The listing builds one solid part. Answer for the finished solid, in the listing's coordinates (mm). Coordinates: 2 decimals unless noted, no trailing zeros. Loops run counter-clockwise (first coordinate to the right, second up) from the corner with the lowest first, then second, coordinate; pieces in that order, holes last. Notation, with made-up numbers: M 25,-15 L 69,-15 A26 ccw 69,17 Z; hole C 14,-13 d5. An arc over 180 degrees is marked long. Return JSON: item names as keys, results as strings. Group by question number.
1. Given P1, Ø1, axis at x = 47.5, z = 345, coming from the -Y side; P2, Ø1, axis at x = 107, z = 347.5, coming from the -Y side, each flat-ended and moving along its own axis, determine where each tip first touches the part or whether it passes through.
2. Section A-A (x = 55) is taken. Write down the section's boundary in (y, z), then the cut area to 3 significant figures.
3. Straight lines are drawn through the part: L1, parallel to X at y = -337.5, z = 346; L2, parallel to X at y = -338.5, z = 343.75; L3, parallel to X at y = -341.5, z = 348.5. For each, find the intervals that lie inside material, in ascending order. Write a range as from..to.
Autodesk Inventor part; units mm, degrees
ref_plane "YZ Plane" through (0, 0, 0) normal (1, 0, 0) x (0, 1, 0)
ref_plane "XZ Plane" through (0, 0, 0) normal (0, 1, 0) x (-1, 0, 0)
ref_plane "XY Plane" through (0, 0, 0) normal (0, 0, 1) x (1, 0, 0)
sketch "Skizze2" plane through (0, 0, 0) normal (1, 0, 0) x (0, 1, 0)
  line L0 (-333.777, 348.0872) -> (-334.0423, 350.6737)
  line L1 (-333.777, 348.0872) -> (-333.134, 341.8201)
  line L2 (-333.134, 341.8201) -> (-342.5844, 340.8506)
  line L3 (-342.0005, 349.8573) -> (-334.0423, 350.6737)
  line L4 (-342.7069, 342.0444) -> (-341.2147, 342.1975)
  line L5 (-342.7069, 342.0444) -> (-342.5844, 340.8506)
  line L6 (-333.134, 341.8201) -> (-342.5844, 340.8506)
  line L7 (-333.777, 348.0872) -> (-333.134, 341.8201)
  line L8 (-333.777, 348.0872) -> (-341.7352, 347.2708)
  line L9 (-341.2147, 342.1975) -> (-341.7352, 347.2708)
  line L10 (-342.7069, 342.0444) -> (-342.5844, 340.8506)
  line L11 (-341.7352, 347.2708) -> (-342.0005, 349.8573)
  point P0 (0, 0)
extrude "Extrusion1" add sketch "Skizze2" along normal blind 69.4
sketch "Skizze3" plane through (0, 0, 0) normal (-1, 0, 0) x (0, 0, 1)
  line L0 (342.0444, -342.7069) -> (342.1975, -341.2147)
  line L1 (342.0444, -342.7069) -> (340.8506, -342.5844)
  line L2 (341.8201, -333.134) -> (340.8506, -342.5844)
  line L3 (348.0872, -333.777) -> (341.8201, -333.134)
  line L4 (348.0872, -333.777) -> (347.2708, -341.7352)
  line L5 (342.1975, -341.2147) -> (347.2708, -341.7352)
  line L6 (350.6737, -334.0423) -> (349.8573, -342.0005)
  line L7 (349.8573, -342.0005) -> (347.2708, -341.7352)
  line L8 (349.8573, -342.0005) -> (342.1975, -341.2147)
  line L9 (341.8201, -333.134) -> (350.6737, -334.0423)
  line L10 (350.6737, -334.0423) -> (348.0872, -333.777)
  point P0 (0, 0)
extrude "Extrusion2" cut sketch "Skizze3" against normal blind 10 contours L4 L9 L6 L7
sketch "Skizze4" plane through (0, -333.134, 341.8201) normal (0, 0.1020498, -0.9947793) x (1, 0, 0)
  line L0 (5, 0) -> (5, 9.5) construction
  line L1 (0, 9.5) -> (69.4, 9.5) construction
  circle A0 centre (5, 4) radius 2.85
  circle A1 centre (5, 4) radius 1.5 construction
  point P0 (0, -296.5122)
  dimension "d4" = 5.7
extrude "Extrusion3" cut sketch "Skizze4" against normal blind 3.1
sketch "Skizze5" plane through (5, -337.4295, 344.4957) normal (0, 0.1020498, -0.9947793) x (-1, 0, 0)
  circle A0 centre (0, 0) radius 2.85
  circle A1 centre (0, 0) radius 1.5
  point P0 (5, 300.5122)
  dimension "d9" = 3
extrude "Extrusion4" cut sketch "Skizze5" against normal blind 3.4 contours A1
mirror "Spiegeln1" about plane through (69.4, -337.8887, 348.9722) normal (1, 0, 0) of "Extrusion4", "Extrusion3", "Extrusion2", "Extrusion1"
properties part number "Case_bottom_front"
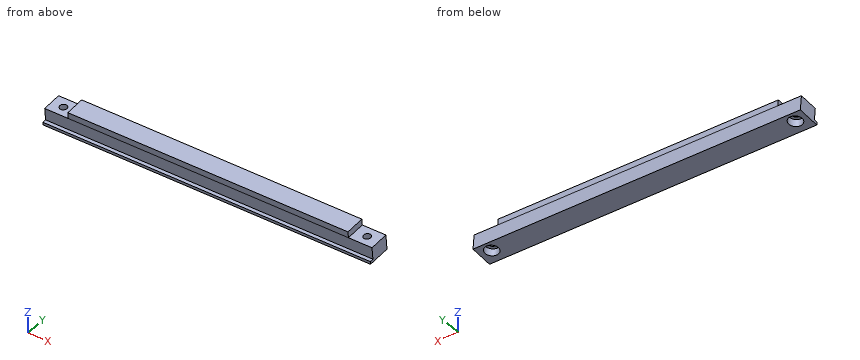
Worked out:
{
 "1": {"P1": "y = -341.55", "P2": "y = -341.81"},
 "2": {"outline": "M -342.71,342.04 L -342.58,340.85 L -333.13,341.82 L -333.78,348.09 L -334.04,350.67 L -342,349.86 L -341.74,347.27 L -341.21,342.2 Z", "area": "73.0 mm^2"},
 "3": {"L1": "0..3.5, 6.5..132.3, 135.3..138.8", "L2": "0..2.39, 7.61..131.19, 136.41..138.8", "L3": "10..128.8"}
}
